Can you work these out from the model? Positions are in its coordinate system, mm. A direction names the side the tool comes from. Coordinates: 2 decimals unless noted, no trailing zeros. Loops run counter-clockwise (first coordinate to the right, second up) from the corner with the lowest first, then second, coordinate; pieces in that order, holes last.
```python
from build123d import *

# Parameters (mm, degrees)
SKETCH_R          = 4.25
PAD_DEPTH         = 28.5
PAD_DEPTH_BACK    = 5
FILLET_R          = 5
SKETCH002_R       = 6.4
POCKET_DEPTH      = 24.001
POCKET_DEPTH_BACK = -16.001
POCKET001_DEPTH   = 3
POCKET002_DEPTH   = 4
POCKET003_DEPTH   = 98.201
POCKET004_DEPTH   = 4
POCKET005_DEPTH   = 16
SKETCH028_R       = 22
POCKET006_DEPTH   = 25
SKETCH031_R       = 2.5
POCKET007_DEPTH   = 9
PAD001_DEPTH      = 17.2
SKETCH034_W       = 50
SKETCH034_H       = 25
POCKET008_DEPTH   = 2
SKETCH036_R       = 4.4
POCKET009_DEPTH   = 1.5
CHAMFER_SIZE      = 1.9
CHAMFER001_SIZE   = 2.5


with BuildPart() as part:
    # Sketch → Pad (new body, two sides)
    with BuildSketch(Plane.XY) as pad_sk:
        with BuildLine():
            ThreePointArc((0, -19), (16, -3), (0, 13))
            Line((0, 44.1), (0, 13))
            ThreePointArc((0, 44.1), (-2.928932, 51.171068), (-10, 54.1))
            Line((-24, 54.1), (-10, 54.1))
            Line((-24, 54.1), (-24, -44.1))
            Line((-24, -44.1), (-1, -44.1))
            ThreePointArc((-1, -44.1), (-0.292893, -43.807107), (0, -43.1))
            Line((0, -19), (0, -43.1))
        make_face()
        with Locations((0, -3)):
            Circle(SKETCH_R, mode=Mode.SUBTRACT)
    extrude(amount=PAD_DEPTH)
    extrude(pad_sk.sketch, amount=-PAD_DEPTH_BACK)

    # Fillet
    fillet_edges = [part.edges().sort_by_distance(p)[0] for p in [
        (0, 13, 11.75),
        (0, -19, 11.75),
    ]]
    fillet(fillet_edges, radius=FILLET_R)

    # Sketch002 → Pocket (cut, two sides)
    with BuildSketch(Plane.YZ) as pocket_sk:
        with Locations((-30, 11.5)):
            Circle(SKETCH002_R)
        with Locations((40, 11.5)):
            Circle(SKETCH002_R)
    extrude(amount=-POCKET_DEPTH, mode=Mode.SUBTRACT)
    extrude(pocket_sk.sketch, amount=-POCKET_DEPTH_BACK, mode=Mode.SUBTRACT)

    # Sketch013 → Pocket001 (cut)
    with BuildSketch(Plane.XY.offset(28.5)):
        with BuildLine():
            ThreePointArc((0, -13), (10, -3), (0, 7))
            Line((-40, 7), (0, 7))
            Line((-40, 7), (-40, 60))
            Line((-40, 60), (30, 60))
            Line((30, 60), (30, -60))
            Line((30, -60), (-40, -60))
            Line((-40, -60), (-40, -13))
            Line((-40, -13), (0, -13))
        make_face()
    extrude(amount=-POCKET001_DEPTH, mode=Mode.SUBTRACT)

    # Sketch024 → Pocket002 (cut)
    with BuildSketch(Plane(origin=(0, 0, -5), x_dir=(1, 0, 0), z_dir=(0, 0, -1))):
        with BuildLine():
            Line((0, 13), (-40, 13))
            Line((-40, 13), (-40, 65))
            Line((-40, 65), (24, 65))
            Line((24, 65), (24, -65))
            Line((24, -65), (-40, -65))
            Line((-40, -7), (-40, -65))
            Line((-40, -7), (0, -7))
            ThreePointArc((0, -7), (10, 3), (0, 13))
        make_face()
    extrude(amount=-POCKET002_DEPTH, mode=Mode.SUBTRACT)

    # Sketch029 → Pocket003 (cut, through all)
    with BuildSketch(Plane(origin=(0, 54.1, 0), x_dir=(-1, 0, 0), z_dir=(0, 1, 0))):
        with BuildLine():
            ThreePointArc((32, 30), (13.221825, 37.778175), (21, 19))
            Line((21, 19), (32, 19))
            Line((32, 30), (32, 19))
        make_face()
    extrude(amount=-POCKET003_DEPTH, mode=Mode.SUBTRACT)

    # Sketch027 → Pocket004 (cut)
    with BuildSketch(Plane(origin=(0, 0, -5), x_dir=(1, 0, 0), z_dir=(0, 0, -1))):
        Polygon((3.925982, 9.8), (-3.925982, 9.8), (-7.851964, 3), (-3.925982, -3.8), (3.925982, -3.8), (7.851964, 3), align=None)
    extrude(amount=-POCKET004_DEPTH, mode=Mode.SUBTRACT)

    # Sketch025 → Pocket005 (cut, symmetric)
    with BuildSketch(Plane.YZ):
        with BuildLine():
            Line((-16, 20.1), (26, 20.1))
            ThreePointArc((30, 16), (28.864001, 18.892928), (26, 20.1))
            Line((30, 16), (30, 7))
            ThreePointArc((26, 2.9), (28.864001, 4.107072), (30, 7))
            Line((26, 2.9), (-16, 2.9))
            ThreePointArc((-20, 7), (-18.864001, 4.107072), (-16, 2.9))
            Line((-20, 7), (-20, 16))
            ThreePointArc((-16, 20.1), (-18.864001, 18.892928), (-20, 16))
        make_face()
    extrude(amount=POCKET005_DEPTH, both=True, mode=Mode.SUBTRACT)

    # Sketch028 → Pocket006 (cut)
    with BuildSketch(Plane(origin=(0, 54.1, 0), x_dir=(-1, 0, 0), z_dir=(0, 1, 0))):
        with Locations((21, -20)):
            Circle(SKETCH028_R)
    extrude(amount=-POCKET006_DEPTH, mode=Mode.SUBTRACT)

    # Sketch031 → Pocket007 (cut)
    with BuildSketch(Plane(origin=(0, 0, -1), x_dir=(1, 0, 0), z_dir=(0, 0, -1))):
        with Locations((-6, 30)):
            Circle(SKETCH031_R)
        with Locations((-6, -40)):
            Circle(SKETCH031_R)
    extrude(amount=-POCKET007_DEPTH, mode=Mode.SUBTRACT)

    # Sketch032 → Pad001 (new body)
    with BuildSketch(Plane.XY.offset(2.9)):
        Polygon((0, -22), (-16, -11.5), (-16, -22), align=None)
        Polygon((-16, 12), (0, 30.1), (-16, 30.1), align=None)
    extrude(amount=PAD001_DEPTH)

    # Sketch034 → Pocket008 (cut)
    with BuildSketch(Plane(origin=(0, 0, -5), x_dir=(1, 0, 0), z_dir=(0, 0, -1))):
        with Locations((-10, 2.5)):
            Rectangle(SKETCH034_W, SKETCH034_H)
    extrude(amount=-POCKET008_DEPTH, mode=Mode.SUBTRACT)

    # Sketch036 → Pocket009 (cut)
    with BuildSketch(Plane(origin=(0, 0, -1), x_dir=(1, 0, 0), z_dir=(0, 0, -1))):
        with Locations((-6, 30)):
            Circle(SKETCH036_R)
        with Locations((-6, -40)):
            Circle(SKETCH036_R)
    extrude(amount=-POCKET009_DEPTH, mode=Mode.SUBTRACT)

    # Chamfer
    chamfer_edges = [part.edges().sort_by_distance(p)[0] for p in [
        (-12, -13, -1),
        (-12, 7, -1),
        (10, -3, -1),
    ]]
    chamfer(chamfer_edges, length=CHAMFER_SIZE)

    # Chamfer001
    chamfer001_edges = [part.edges().sort_by_distance(p)[0] for p in [
        (10, -3, 25.5),
        (-5.481285, -13, 25.5),
        (-5.481285, 7, 25.5),
    ]]
    chamfer(chamfer001_edges, length=CHAMFER001_SIZE)


solid = part.part
```
Item 1: Suppose I cut it at B-B, the plane z = 11.5. Please give me the cut outline in (x, y).
Results are:
outline: (-24, -44.1) - (-1, -44.1) arc R1 ccw to (0, -43.1) - (0, -36.4) - (-24, -36.4) - close; (-24, -23.6) - (0, -23.6) - (0, -23.4) arc R5 cw to (1.33, -20) - (-3.05, -20) - (-16, -11.5) - (-16, 12) - (-0.09, 30) - (0, 30) - (0, 33.6) - (-24, 33.6) - close; (-24, 46.4) - (-0.27, 46.4) arc R10 ccw to (-10, 54.1) - (-24, 54.1) - close
Item 2: I need wall thicknesses on line 1 along Y through (x, z) = (-6, 2); line 2 along Z through (x, y) = (-3.5, 15); line 3 along Y through (x, z) = (-9, 11). Which ranges of each line are inside material? Lowest first, please.
Results are:
line 1: y = -44.1 to -32.5, -27.5 to 37.5, 42.5 to 53.27
line 2: z = -1 to 2.9, 20.1 to 25.5
line 3: y = -44.1 to -36.38, -23.62 to -16.09, 19.92 to 33.62, 46.38 to 54.05
Item 3: Suppose I cut it at A-A, the plane y = -30. Please give me the cut outline in (x, z), plus the area to 3 significant figures.
Results are:
outline: (-24, -1) - (-10.4, -1) - (-10.4, 0.5) - (-8.5, 0.5) - (-8.5, 5.1) - (-24, 5.1) - close; (-24, 17.9) - (0, 17.9) - (0, 25.5) - (-10.96, 25.5) arc R11 cw to (-21, 19) - (-24, 19) - close; (-3.5, 0.5) - (-1.6, 0.5) - (-1.6, -1) - (0, -1) - (0, 5.1) - (-3.5, 5.1) - close
area: 226 mm2
Item 4: We'd pull the mould along Z, two halves only. Please class faces 4 (the face through (-3.3, 0, 20.1)), 5 (the face through (-6.33, 37.52, 3.02)), 6 (the face through (-16.82, 41.78, 1.6)): +Z half, -Z half, draft (parallel to the pull), parting line (faces both ways), or undercut.
Results are:
face 4: undercut
face 5: draft
face 6: -Z half
Item 5: On a 3-axis mill with a long thin cutter (end or side, diameter ignored), from which of +Z, -Z, +X, -X, +Y, -Y can I reach the whole of each face in a straight line? I mean faces 1 (the face through (-8.16, 20.87, 11.38)), 2 (the face through (0, -9.8, -2)), 3 (the face through (0, -35.3, 15.4)). Say none if no direction works.
Results are:
face 1: +X
face 2: -Z
face 3: +Z, -Z, +X, -Y
Item 6: I'm going to push flat-ended pins straight in: P1, Ø9.5, axis at x = -5.5, y = -30.5, coming from the -Z side; P2, Ø6, axis at x = -16.5, y = -30.5, coming from the +Z side; P3, Ø8.5, axis at y = 4, z = 13, coming from the +X side; P4, Ø12, axis at x = -5.5, z = 18, coming from the +Y side. Where does each tip first touch, or does it pass through?
Results are:
P1: stops at z = -1
P2: stops at z = 21.95
P3: stops at x = -16
P4: stops at y = 54.1
Item 7: Suppose I cut it at D-D, the plane y = 40. Please give me the cut outline in (x, z).
Results are:
outline: (-24, 1.79) arc R22 cw to (-10.4, -0.72) - (-10.4, 0.5) - (-8.5, 0.5) - (-8.5, 5.1) - (-24, 5.1) - close; (-24, 17.9) - (0, 17.9) - (0, 25.5) - (-10.96, 25.5) arc R11 cw to (-21, 19) - (-24, 19) - close; (-3.5, 0.5) - (-1.6, 0.5) - (-1.6, -1) - (0, -1) - (0, 5.1) - (-3.5, 5.1) - close
Item 8: Suppose I cut it at C-C, the plane x = -17. Please give me the cut outline in (y, z).
Results are:
outline: (-44.1, -1) - (-14.9, -1) - (-13, -2.9) - (-13, -3) - (7, -3) - (7, -2.9) - (8.9, -1) - (29.1, -1) - (29.1, 1.63) - (54.1, 1.63) - (54.1, 19.75) - (-44.1, 19.75) - close; hole circle Ø12.8 at (-30, 11.5); hole circle Ø12.8 at (40, 11.5)
